Here's how the part is built. I have some questions about the finished solid (model axes, mm). Coordinates: 2 decimals unless noted, no trailing zeros. Order: outer loops, then holes, each group sorted by start corner. A loop starts at its lowest first (then second) coordinate and runs counter-clockwise, first axis right, second up. Notation, with made-up numbers: (-17, -15) - (15, -15) arc R7 ccw to (15, -3) - close; hole circle Ø3 at (-8, 76). An arc over 180 degrees is marked (long way). Use CSV: the item, a comma, the result in double quotes. Start each with the question number.
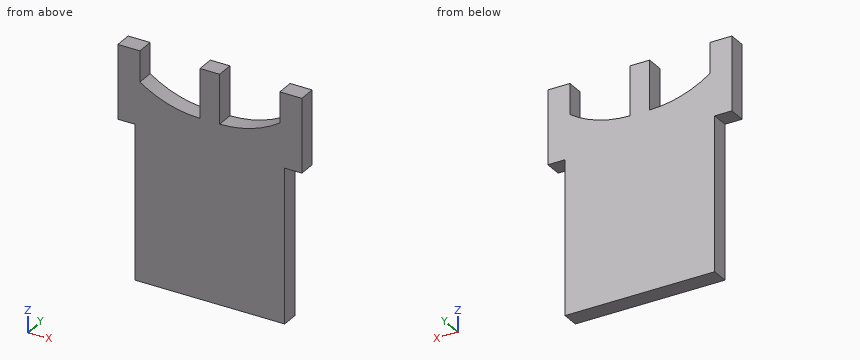
from build123d import *

# Parameters (mm, degrees)
F1_DEPTH = 14


with BuildPart() as f1:
    # F0 (on Front) → F1 (new body)
    with BuildSketch(Plane.XZ):
        with BuildLine():
            Line((0, 185), (0, 0))
            Line((0, 0), (61, 0))
            Line((61, 0), (61, 125))
            Line((61, 125), (75, 125))
            Line((75, 125), (75, 185))
            Line((75, 185), (57, 185))
            Line((57, 185), (57, 160))
            ThreePointArc((57, 160), (33.622256, 148.833964), (8, 145))
            Line((8, 145), (8, 185))
            Line((8, 185), (0, 185))
        make_face()
        with BuildLine():
            Line((-61, 125), (-61, 0))
            Line((-61, 0), (0, 0))
            Line((0, 0), (0, 185))
            Line((0, 185), (-8, 185))
            Line((-8, 185), (-8, 145))
            ThreePointArc((-8, 145), (-33.622256, 148.833964), (-57, 160))
            Line((-57, 160), (-57, 185))
            Line((-57, 185), (-75, 185))
            Line((-75, 185), (-75, 125))
            Line((-75, 125), (-61, 125))
        make_face()
    extrude(amount=F1_DEPTH)


solid = f1.part
Item 1: Suppose I cut it at B-B on y = -3.5. Write out the boundary of the cut face in (x, z), then the cut area to 3 significant figures.
Item 2: For pin 1 Ø3 at (x, y) = (42.5, -3.5) entering from -Z; pin 2 Ø7 at (x, y) = (71.5, -10) entering from -Z; pin 3 Ø2 at (y, z) = (-6, 118.5) entering from +X; pin 4 Ø6 at (y, z) = (-6, 72.5) entering from -X, each with a flat end and sliding along its axis, tell me the tip position at first contact or that it passes through.
Item 3: Suppose I cut it at A-A on z = 167. Write out the boundary of the cut face in (x, y), then the cut area to 3 significant figures.
Item 4: Please list where these lines run through material, in increasing order: line 1 along X through (y, z) = (-4.25, 160); line 2 along X through (y, z) = (-3.5, 152); line 3 along Z through (x, y) = (-62, -1). Write a range as from..to.
Item 5: Suppose I cut it at C-C on x = 17. Write out the boundary of the cut face in (y, z), then the cut area to 3 significant figures.
Item 6: Suppose I cut it at D-D on z = 86.5. Write out the boundary of the cut face in (x, y), then the cut area to 3 significant figures.
Here are the results:
1,outline,"(-75, 125) - (-61, 125) - (-61, 0) - (61, 0) - (61, 125) - (75, 125) - (75, 185) - (57, 185) - (57, 160) arc R87.53 cw to (8, 145) - (8, 185) - (-8, 185) - (-8, 145) arc R87.53 cw to (-57, 160) - (-57, 185) - (-75, 185) - close"
1,area,"20,800 mm^2"
2,pin 1,"z = 0"
2,pin 2,"z = 125"
2,pin 3,"x = 61"
2,pin 4,"x = -61"
3,outline,"(-75, -14) - (-57, -14) - (-57, 0) - (-75, 0) - close; (-8, -14) - (8, -14) - (8, 0) - (-8, 0) - close; (57, -14) - (75, -14) - (75, 0) - (57, 0) - close"
3,area,"728 mm^2"
4,line 1,"-75..-57, -8..8, 57..75"
4,line 2,"-75..-42.3, -8..8, 42.3..75"
4,line 3,"125..185"
5,outline,"(-14, 0) - (0, 0) - (0, 145.46) - (-14, 145.46) - close"
5,area,"2,040 mm^2"
6,outline,"(-61, -14) - (61, -14) - (61, 0) - (-61, 0) - close"
6,area,"1,710 mm^2"
